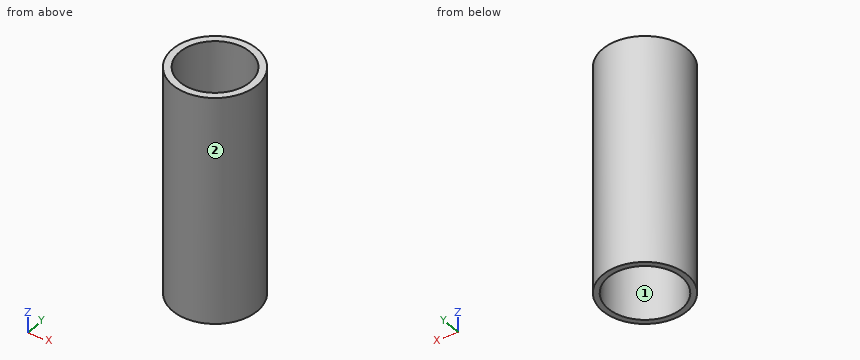
from build123d import *

# Parameters (mm, degrees)
F0_R     = 7.625
F0_R_2   = 6.625
F1_DEPTH = 20
F2_R     = 7.625
F2_R_2   = 6.625
F2_R_3   = 3.625
F3_DEPTH = 1.1
F4_R     = 7.625
F4_R_2   = 6.35
F5_DEPTH = 20


with BuildPart() as f1:
    # F0 (on Top) → F1 (new body)
    with BuildSketch(Plane.XY):
        Circle(F0_R)
        Circle(F0_R_2, mode=Mode.SUBTRACT)
    extrude(amount=F1_DEPTH)

    # F2 (on face) → F3 (join)
    with BuildSketch(Plane.XY.offset(20)):
        Circle(F2_R)
        Circle(F2_R_2, mode=Mode.SUBTRACT)
        Circle(F2_R_2)
        Circle(F2_R_3, mode=Mode.SUBTRACT)
    extrude(amount=F3_DEPTH)

    # F4 (on face) → F5 (join)
    with BuildSketch(Plane.XY.offset(21.1)):
        Circle(F4_R)
        Circle(F4_R_2, mode=Mode.SUBTRACT)
    extrude(amount=F5_DEPTH)


solid = f1.part
Check sheet for the modelled part. Datum: model origin and axes. Units: mm. Face numbers are marked on the shaded views. Round coordinates to 2 decimals unless told otherwise and drop trailing zeros. Loops run counter-clockwise (first coordinate to the right, second up) from the corner with the lowest first, then second, coordinate; pieces in that order, holes last. Notation, with made-up numbers: M -28.75,-12 L 9.25,-12 A26 cw 9.25,12 Z; hole C 77.25,79.25 d3. An arc over 180 degrees is marked long. One line per question, with ' | ' between items. Start each with the question number.
Item 1: Section check A-A (y = 0). Record the boundary of the cut face in (x, z) (3 decimals), and give its area (3 significant figures).
Item 2: Section check D-D (z = 22). Record the boundary of the cut face in (x, y) (3 decimals).
Item 3: Gauge pin test, flat ends, axial feed: pin 1 Ø2 at (x, z) = (-3.5, 21.5) entering from -Y; pin 2 Ø1.5 at (y, z) = (5.5, 7.5) entering from -X; pin 3 Ø6 at (x, y) = (0, 0) entering from +Z; pin 4 Ø4 at (x, z) = (3.5, 35.5) entering from +Y. Record the tip position at first contact, or that the pin passes through.
Item 4: Scan lines: probe 1 along Y at (x, z) = (0, 20.35) (3 decimals); probe 2 along Y at (x, z) = (-1.5, 38); probe 3 along Z at (x, y) = (3.75, 3.75). Record each from-to range of solid material in increasing order.
Item 5: Release check for a two-part mould opening along Y. For the marked faces 1 and 2 record: released by +Y, released by -Y, zero draft, split by the parting line, or undercut.
Item 6: Section check C-C (z = 7.5). Record the boundary of the cut face in (x, y) (3 decimals), and give its area (3 significant figures).
Worked out:
1) outline: M -7.625,0 L -6.625,0 L -6.625,20 L -3.625,20 L -3.625,21.1 L -6.35,21.1 L -6.35,41.1 L -7.625,41.1 Z; M 3.625,20 L 6.625,20 L 6.625,0 L 7.625,0 L 7.625,41.1 L 6.35,41.1 L 6.35,21.1 L 3.625,21.1 Z | area: 99.8 mm^2
2) outline: C 0,0 d15.25; hole C 0,0 d12.7
3) pin 1: y = -7.2 | pin 2: x = -5.96 | pin 3: through | pin 4: y = 7.48
4) probe 1: -7.625 to -3.625, 3.625 to 7.625 | probe 2: -7.48 to -6.17, 6.17 to 7.48 | probe 3: 20 to 21.1
5) face 1: undercut | face 2: split by the parting line
6) outline: C 0,0 d15.25; hole C 0,0 d13.25 | area: 44.8 mm^2
